Part model, mm, in its own coordinate system. Face numbers are marked on the shaded views. A direction names the side the tool comes from. Coordinates: 2 decimals unless noted, no trailing zeros. Order: outer loops, then holes, each group sorted by start corner. A loop starts at its lowest first (then second) coordinate and runs counter-clockwise, first axis right, second up.
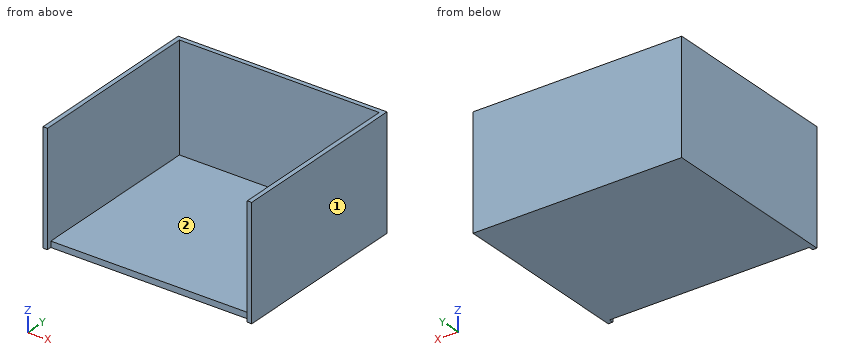
from build123d import *

# Parameters (mm, degrees)
F0_W     = 800
F0_H     = 700
F1_DEPTH = 24
F2_W     = 18
F2_H     = 736
F3_DEPTH = 450
F4_W     = 800
F4_H     = 18
F6_DEPTH = 450


with BuildPart() as f1:
    # F0 (on Top) → F1 (new body)
    with BuildSketch(Plane.XY):
        Rectangle(F0_W, F0_H)
    extrude(amount=F1_DEPTH)

    # F2 (on Top) → F3 (join)
    with BuildSketch(Plane.XY):
        with Locations((409, 0)):
            Rectangle(F2_W, F2_H)
    extrude(amount=F3_DEPTH)

    # F5: F1 across plane


with BuildPart() as f1_1:
    add(f1.part)
    add(f1.part.mirror(Plane.YZ))

    # F4 (on Top) → F6 (join)
    with BuildSketch(Plane.XY):
        with Locations((0, 359)):
            Rectangle(F4_W, F4_H)
    extrude(amount=F6_DEPTH)


solid = f1_1.part
Q1. Wall check: line 1 along X through (y, z) = (-274.5, 392.5); line 2 along Y through (x, z) = (159, 148.5); line 3 along Z through (x, y) = (367.5, -155). Give the ranges that are in metal, low to high.
Results list:
line 1: x = -418 to -400, 400 to 418
line 2: y = 350 to 368
line 3: z = 0 to 24
Q2. Cut at A-A on z = 117.5. Write the cut outline in (x, y), and give its area (3 significant figures).
Results list:
outline: (-418, -368) - (-400, -368) - (-400, 350) - (400, 350) - (400, -368) - (418, -368) - (418, 368) - (-418, 368) - close
area: 40,900 mm2
Q3. Pin check, flat tips, straight feed: pin 1 Ø5 at (x, y) = (-65, 263.5) entering from +Z; pin 2 Ø10 at (x, z) = (-60, 240.5) entering from -Y. Stop position of each tip, or through.
Results list:
pin 1: stops at z = 24
pin 2: stops at y = 350
Q4. Cut at B-B on y = -244. Write the cut outline in (x, z), and give its area (3 significant figures).
Results list:
outline: (-418, 0) - (418, 0) - (418, 450) - (400, 450) - (400, 24) - (-400, 24) - (-400, 450) - (-418, 450) - close
area: 35,400 mm2
Q5. Cut at C-C on x = 25. Write the cut outline in (y, z), and give its area (3 significant figures).
Results list:
outline: (-350, 0) - (368, 0) - (368, 450) - (350, 450) - (350, 24) - (-350, 24) - close
area: 24,900 mm2
Q6. Which spindle directions (+Z, -Z, +X, -X, +Y, -Y) get a long thin tool onto all of the face, cutting with end or side? Do the marked faces 1 and 2. Say none if no direction does.
Results list:
face 1: +Z, -Z, +X, +Y, -Y
face 2: +Z, -Y
